Here's the drawing with two shaded views (mm, measured from the low corner). I have some questions. A direction names the side the tool comes from. Give positions to 0.01 mm unless a question says otherwise; leave off trailing zeros. Write each loop counter-clockwise with the first axis right and the second up, starting at its lowest first coordinate (ties: lowest second). Pieces come first, ordered by that corner, then holes. Notation, with made-up numbers: (72.5, 23) - (83.5, 23) arc R26 ccw to (83.5, 47) - close; hole circle Ø11 at (-0.75, 50.5). An arc over 180 degrees is marked (long way). Answer as CSV lines item,"result". Start each with the question number.
Q1. Imagine slicing it at C-C on y = 20.5. List the corners of the cut face in (x, z) for me, and give its area (3 significant figures).
Q2. On a 3-axis mill with a long thin cutter (end or side, diameter ignored), from which of +Z, -Z, +X, -X, +Y, -Y can I reach the whole of each face in a straight line? I mean the marked faces 1 and 2. Say none if no direction works.
Q3. Will these pins go through, and if not, where does the flat tip stop? pin 1 Ø15 at (x, y) = (26, 35) entering from -Z; pin 2 Ø6 at (x, z) = (33.5, 6.5) entering from +Y; pin 3 Ø6 at (x, z) = (7.5, 18.5) entering from +Y; pin 4 Ø4 at (y, z) = (40.5, 26) entering from +X.
Q4. Imagine slicing it at D-D on y = 14.5. List the corners of the cut face in (x, z) for me, and give its area (3 significant figures).
Q5. Imagine slicing it at A-A on x = 25.4. List the corners of the cut face in (y, z) for me.
Q6. If I drill on line 1 along Y through (x, z) = (25, 10); line 2 along Z through (x, y) = (16, 43.5), over which ranges is the centre line in solid material (lowest first)?
Q7. We'd pull the mould along Z, two halves only. Please class the marked faces 3, 4 and 5: pulls with the +Z half, pulls with the -Z half, needs draft (parallel to the pull), parting line crosses it, or undercut.
Q8. Imagine slicing it at B-B on z = 22.5. List the corners of the cut face in (x, y) for me, and give its area (3 significant figures).
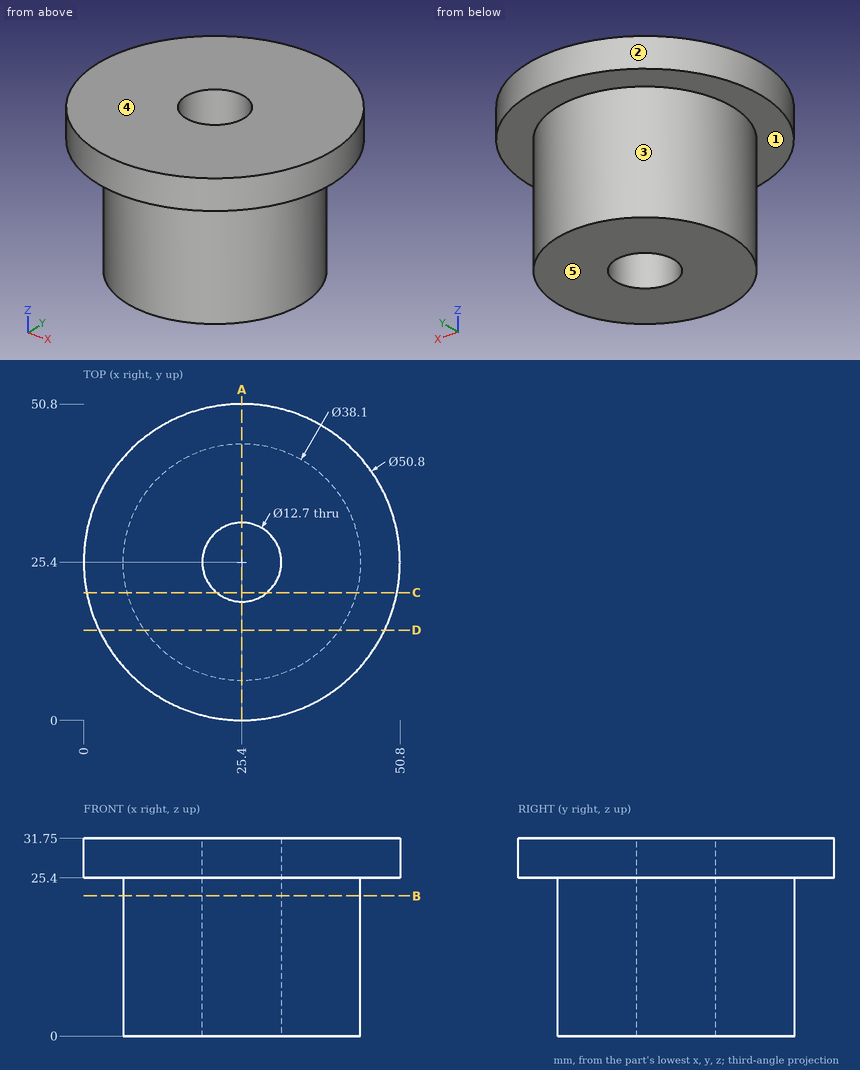
Conclusion:
1,outline,"(0.48, 25.4) - (6.99, 25.4) - (6.99, 0) - (21.36, 0) - (21.36, 31.75) - (0.48, 31.75) - close; (29.44, 0) - (43.81, 0) - (43.81, 25.4) - (50.32, 25.4) - (50.32, 31.75) - (29.44, 31.75) - close"
1,area,"995 mm^2"
2,face 1,"-Z"
2,face 2,"+Z, -Z"
3,pin 1,"z = 0"
3,pin 2,"y = 43.75"
3,pin 3,"y = 37.27"
3,pin 4,"x = 47.16"
4,outline,"(2.46, 25.4) - (9.78, 25.4) - (9.78, 0) - (41.02, 0) - (41.02, 25.4) - (48.34, 25.4) - (48.34, 31.75) - (2.46, 31.75) - close"
4,area,"1,090 mm^2"
5,outline,"(0, 25.4) - (6.35, 25.4) - (6.35, 0) - (19.05, 0) - (19.05, 31.75) - (0, 31.75) - close; (31.75, 0) - (44.45, 0) - (44.45, 25.4) - (50.8, 25.4) - (50.8, 31.75) - (31.75, 31.75) - close"
6,line 1,"6.35 to 19.06, 31.74 to 44.45"
6,line 2,"25.4 to 31.75"
7,face 3,"needs draft"
7,face 4,"pulls with the +Z half"
7,face 5,"pulls with the -Z half"
8,outline,"circle Ø38.1 at (25.4, 25.4); hole circle Ø12.7 at (25.4, 25.4)"
8,area,"1,010 mm^2"
